from build123d import *

# Parameters (mm, degrees)
SKETCH_1_W          = 74.6
SKETCH_1_H          = 5
EXTRUDE_1_DEPTH     = 10
SKETCH_4_W          = 10
SKETCH_4_H          = 10
EXTRUDE_2_DEPTH     = 3.5
FILLET_1_R          = 5
SKETCH_2_R          = 2.15
SKETCH_2_R_2        = 1.1
CUT_EXTRUDE_1_DEPTH = 40.541623639


with BuildPart() as part:
    # 스케치1 → 보스-돌출1 (new body)
    with BuildSketch(Plane.XY):
        Rectangle(SKETCH_1_W, SKETCH_1_H)
    extrude(amount=EXTRUDE_1_DEPTH)

    # 스케치4 → 보스-돌출2 (add)
    with BuildSketch(Plane(origin=(0, 2.5, 0), x_dir=(1, 0, 0), z_dir=(0, 1, 0))):
        with Locations((-32.3, -5)):
            Rectangle(SKETCH_4_W, SKETCH_4_H)
    extrude(amount=EXTRUDE_2_DEPTH)

    # 필렛1
    fillet_1_edges = [part.edges().sort_by_distance(p)[0] for p in [
        (37.3, 0, 0),
        (37.3, 0, 10),
        (-37.3, 1.75, 0),
        (-37.3, 1.75, 10),
        (-27.3, 4.25, 10),
        (-27.3, 4.25, 0),
    ]]
    fillet(fillet_1_edges, radius=FILLET_1_R - 0.0001)  # a hair under: the kernel refuses the full size

    # 스케치2 → 컷-돌출1 (cut, through all)
    with BuildSketch(Plane(origin=(0, 6, 0), x_dir=(1, 0, 0), z_dir=(0, 1, 0))):
        with Locations(Location((-32.3, -5, 0), (0, 0, 270))):
            Circle(SKETCH_2_R)
        with Locations(Location((32.3, -5, 0), (0, 0, 270))):
            Circle(SKETCH_2_R_2)
        with Locations(Location((23.3, -5, 0), (0, 0, 270))):
            Circle(SKETCH_2_R_2)
        with Locations(Location((9.3, -5, 0), (0, 0, 270))):
            Circle(SKETCH_2_R_2)
        with Locations(Location((0.3, -5, 0), (0, 0, 270))):
            Circle(SKETCH_2_R_2)
    extrude(amount=-CUT_EXTRUDE_1_DEPTH, mode=Mode.SUBTRACT)


solid = part.part
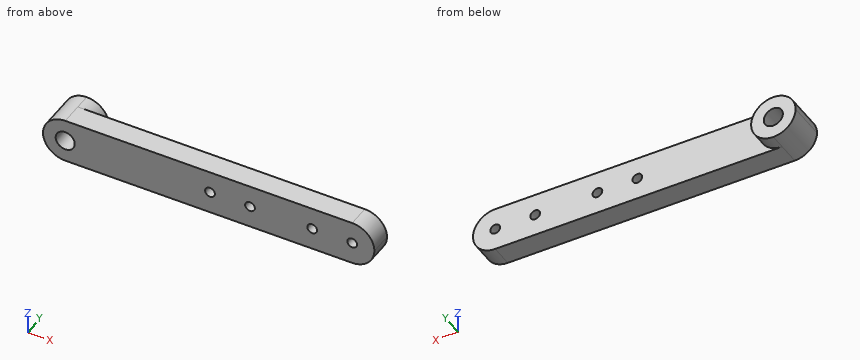
Can you work these out from the model? Positions are in its coordinate system, mm. Coordinates: 2 decimals unless noted, no trailing zeros. Write each loop counter-clockwise with the first axis right and the second up, starting at its lowest first coordinate (ties: lowest second). Pieces come first, ordered by that corner, then holes. Notation, with made-up numbers: M 85.25,65 L 94.25,65 A38 cw 94.25,104 Z; hole C 82.5,-39.5 d7. An arc over 180 degrees is marked long. Use one line per item in the form item = value.
Q1. For P1, Ø1.5, axis at y = 1, z = 6.5, coming from the -X side; P2, Ø4, axis at x = -13.5, z = 2.5, coming from the +Y side; P3, Ø1.5, axis at y = 1.5, z = 2.5, coming from the +X side, each with a flat end and sliding along its axis, tell me the tip position at first contact or that it passes through.
Model answer:
P1 = -37.24
P2 = 2.5
P3 = 36.98
Q2. If we section it at A-A (x = 0.3): Write out the boundary of the cut face in (y, z), then the cut area to 3 significant figures.
Model answer:
outline = M -2.5,0 L 2.5,0 L 2.5,3.9 L -2.5,3.9 Z; M -2.5,6.1 L 2.5,6.1 L 2.5,10 L -2.5,10 Z
area = 39.0 mm^2
Q3. If we section it at B-B (y = 0.25): State how many separate pieces and enclosed holes the cut face has, then the cut area to 3 significant figures.
Model answer:
separate_pieces = 1
enclosed_holes = 5
area = 695 mm^2
Q4. I need wall thicknesses on line 1 along X through (y, z) = (0.3, 5); line 2 along X through (y, z) = (0.75, 4.5); line 3 along Y through (x, z) = (21, 6.5). Which ranges of each line are inside material? Lowest first, please. Write a range as from..to.
Model answer:
line_1 = -37.3..-34.45, -30.15..-0.8, 1.4..8.2, 10.4..22.2, 24.4..31.2, 33.4..37.3
line_2 = -37.27..-34.39, -30.21..-0.68, 1.28..8.32, 10.28..22.32, 24.28..31.32, 33.28..37.27
line_3 = -2.5..2.5
